The model under review builds one solid part; all positions refer to its coordinate system, in mm. Face numbers are marked on the shaded views. Give positions to 0.01 mm unless a question says otherwise; leave off trailing zeros. Loops run counter-clockwise (first coordinate to the right, second up) from the corner with the lowest first, then second, coordinate; pieces in that order, holes last. Notation, with made-up numbers: (71, 10.25) - (117, 10.25) arc R23 ccw to (117, 24.25) - close; hole circle Ø5 at (88, 39). An arc over 180 degrees is marked (long way). Return JSON: item names as keys, results as strings. Group by question number.
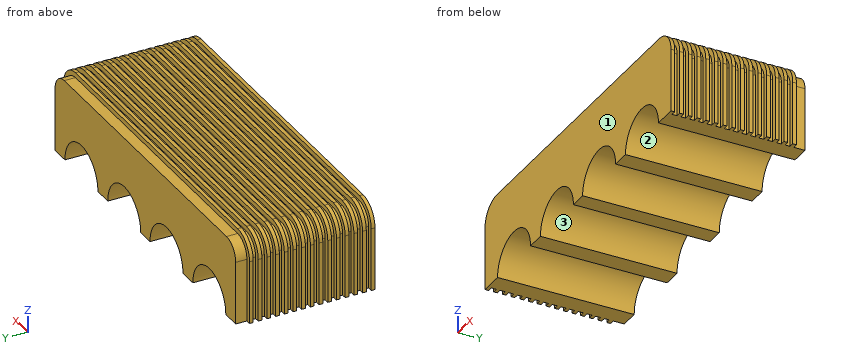
from build123d import *

# Parameters (mm, degrees)
BOSS_EXTRUDE1_DEPTH = 110
BOSS_EXTRUDE2_DEPTH = 3
LPATTERN5_COUNT     = 15
LPATTERN5_PITCH     = 7


with BuildPart() as part:
    # Sketch1 → Boss-Extrude1 (new body)
    with BuildSketch(Plane(origin=(0, 0, 0), x_dir=(1, 0, 0), z_dir=(0, 1, 0))):
        with BuildLine():
            ThreePointArc((57, 0), (32, -25), (7, 0))
            Line((7, 0), (-7, 0))
            ThreePointArc((-7, 0), (-32, -25), (-57, 0))
            Line((-57, 0), (-72, 0))
            ThreePointArc((-72, 0), (-97, -25), (-122, 0))
            Line((-122, 0), (-137, 0))
            Line((-137, 0), (-137, -51))
            ThreePointArc((-137, -51), (-132.899494937, -60.899494937), (-123, -65))
            Line((-123, -65), (123, -65))
            ThreePointArc((123, -65), (132.899494937, -60.899494937), (137, -51))
            Line((137, -51), (137, 0))
            Line((137, 0), (122, 0))
            ThreePointArc((122, 0), (97, -25), (72, 0))
            Line((72, 0), (57, 0))
        make_face()
    extrude(amount=BOSS_EXTRUDE1_DEPTH)

    # Sketch2 → Boss-Extrude2 (add)
    with BuildSketch(Plane.XZ):
        with BuildLine():
            Line((123, 69), (-123, 69))
            ThreePointArc((-123, 69), (-135.727922061, 63.727922061), (-141, 51))
            Line((-141, 51), (-141, 0))
            Line((-141, 0), (-137, 0))
            Line((-137, 0), (-137, 51))
            ThreePointArc((-137, 51), (-132.899494937, 60.899494937), (-123, 65))
            Line((-123, 65), (123, 65))
            ThreePointArc((123, 65), (132.899494937, 60.899494937), (137, 51))
            Line((137, 51), (137, 0))
            Line((137, 0), (141, 0))
            Line((141, 0), (141, 51))
            ThreePointArc((141, 51), (135.727922061, 63.727922061), (123, 69))
        make_face()
    boss_extrude2 = extrude(amount=-BOSS_EXTRUDE2_DEPTH)

    # LPattern5: Boss-Extrude2 ×15
    with Locations(*[(0, i * LPATTERN5_PITCH, 0) for i in range(1, LPATTERN5_COUNT)]):
        add(boss_extrude2)


solid = part.part
Item 1: Take a section at B-B (z = 7). State how many separate pieces and enclosed holes the cut face has, then the cut area to 3 significant figures.
Item 2: Take a section at A-A (y = 103.5). State the section outline as (x, z) points.
Item 3: Mouldability with a two-part tool opening along X and no side actions: class the marked faces 1, 2 and 3 as +X half, -X half, draft (parallel to the pull), parting line (faces both ways), or undercut.
Item 4: For L1, parallel to X at y = 7.5, z = 6.5; L2, parallel to X at y = 11, z = 16; L3, parallel to Z at x = -124, y = 105, list the stretches that pass through material, from the lowest coordinate up. Write a range as from..to.
Item 5: For P1, Ø2, axis at x = 47.5, y = 19.5, coming from the +Z side; P2, Ø1.2, axis at y = 74.5, z = 13.5, coming from the -X side; P3, Ø4, axis at x = -31.5, y = 81, coming from the -Z side, all flat-tipped, find the tip position at first contact; note any pin that passes through.
Check sheet entries:
{
 "1": {"separate pieces": "5", "enclosed holes": "0", "area": "9,380 mm^2"},
 "2": {"outline": "(-137, 0) - (-122, 0) arc R25 cw to (-72, 0) - (-57, 0) arc R25 cw to (-7, 0) - (7, 0) arc R25 cw to (57, 0) - (72, 0) arc R25 cw to (122, 0) - (137, 0) - (137, 51) arc R14 ccw to (123, 65) - (-123, 65) arc R14 ccw to (-137, 51) - close"},
 "3": {"face 1": "draft", "face 2": "undercut", "face 3": "undercut"},
 "4": {"L1": "x = -141..-121.14, -72.86..-56.14, -7.86..7.86, 56.14..72.86, 121.14..141", "L2": "x = -137..-116.21, -77.79..-51.21, -12.79..12.79, 51.21..77.79, 116.21..137", "L3": "z = 0..64.96"},
 "5": {"P1": "stops at z = 65", "P2": "stops at x = -137", "P3": "stops at z = 24.87"}
}
